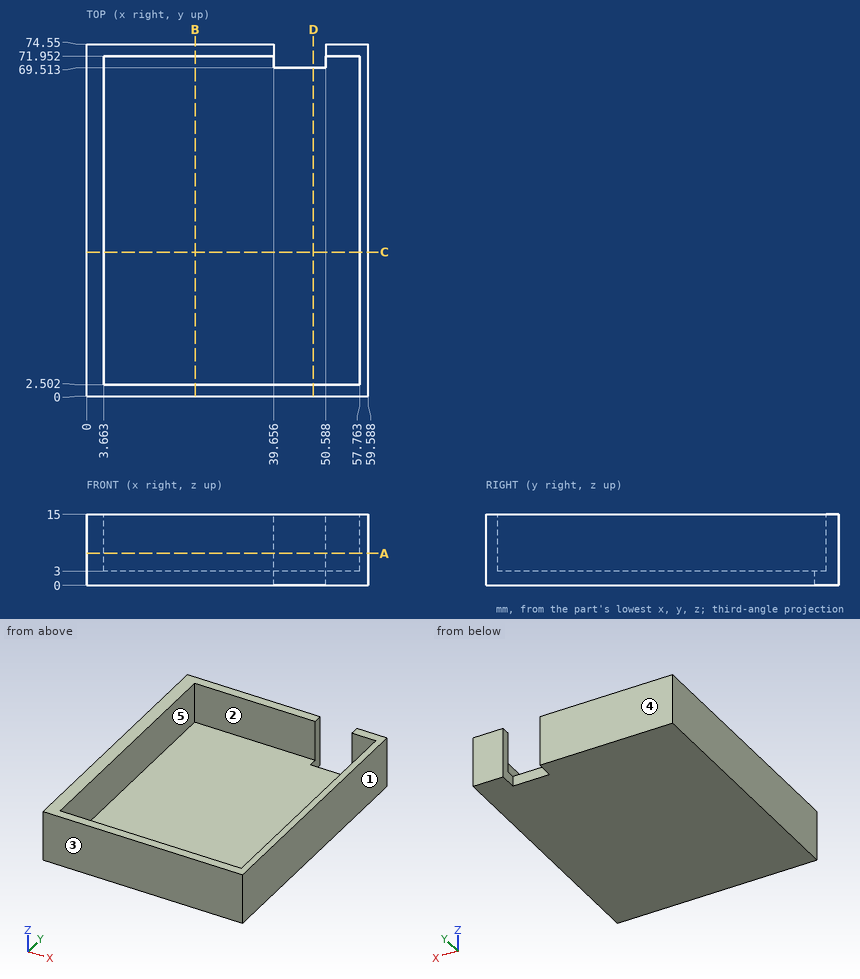
Part print with two shaded views. Sizes in mm from the minimum x, y, z corner. A direction names the side the tool comes from. Give positions to 0.01 mm unless a question says otherwise; leave off trailing zeros. Order: outer loops, then holes, each group sorted by start corner. A loop starts at its lowest first (then second) coordinate and runs counter-clockwise, first axis right, second up.
(1) Saw through at B-B, the plane x = 23. Give the cut face in (y, z), then the cut area to 3 significant figures.
(2) Saw through at A-A, the plane z = 6.75. Give the cut face in (x, y).
(3) Tool access for the marked faces 4 and 5: list every direction of +Z, -Z, +X, -X, +Y, -Y with a clear straight run to the whole face (end or side of a thin tool).
(4) Mould opens along X. For the marked faces 1, 2 and 3 say: released by +X, released by -X, zero draft, split by the parting line, or undercut.
(5) Drill centre lines: L1, parallel to X at y = 65, z = 11.5; L2, parallel to Y at x = 54, z = 8.25; L3, parallel to Y at x = 48.5, z = 13. Where is each one in solid material? Low to high.
(6) Saw through at D-D, the plane x = 48. Give the cut face in (y, z).
(7) Flat gauge pins, fed straight in: pin 1 (1.5 mm diameter, centred on x = 24.5, y = 49, fed in from +Z); pin 2 (6 mm diameter, centred on x = 44.5, z = 6.5, fed in from +Y); pin 3 (2.5 mm diameter, centred on x = 44, z = 1, fed in from +Y). Where does each tip first touch, or does it go through?
(8) Saw through at C-C, the plane y = 30.5. Give the cut face in (x, z).
Results found:
1. outline: (0, 0) - (74.55, 0) - (74.55, 15) - (71.95, 15) - (71.95, 3) - (2.5, 3) - (2.5, 15) - (0, 15) - close
1. area: 285 mm2
2. outline: (0, 0) - (59.59, 0) - (59.59, 74.55) - (50.59, 74.55) - (50.59, 71.95) - (57.76, 71.95) - (57.76, 2.5) - (3.66, 2.5) - (3.66, 71.95) - (39.66, 71.95) - (39.66, 74.55) - (0, 74.55) - close
3. face 4: +Z, -Z, +X, -X, +Y
3. face 5: +Z
4. face 1: released by +X
4. face 2: undercut
4. face 3: zero draft
5. L1: x = 0 to 3.66, 57.76 to 59.59
5. L2: y = 0 to 2.5, 71.95 to 74.55
5. L3: y = 0 to 2.5
6. outline: (0, 0) - (69.51, 0) - (69.51, 3) - (2.5, 3) - (2.5, 15) - (0, 15) - close
7. pin 1: stops at z = 3
7. pin 2: stops at y = 2.5
7. pin 3: stops at y = 69.51
8. outline: (0, 0) - (59.59, 0) - (59.59, 15) - (57.76, 15) - (57.76, 3) - (3.66, 3) - (3.66, 15) - (0, 15) - close
